CAD build for the part. Positions are in the model's coordinates, mm. Face numbers are marked on the shaded views. A direction names the side the tool comes from. Give positions to 0.01 mm unless a question says otherwise; leave off trailing zeros. Order: outer loops, then holes, each group sorted by start corner. A loop starts at its lowest first (then second) coordinate and runs counter-clockwise, first axis right, second up. Notation, with made-up numbers: (44.5, 52) -> (62.5, 52) arc R33 ccw to (62.5, 84) -> close; hole circle Ø4 at (29.25, 2). An arc over 180 degrees is marked (long way). Use one line per item in the form item = value. Start each with the question number.
1) Drop flat-ended pins along their axis: P1, Ø12, axis at y = -218.5, z = -138.5, coming from the -X side; P2, Ø8, axis at y = -97.5, z = -104.5, coming from the +X side. Give the stop position or say it passes through.
2) Tool access for the marked faces 4, 5, 6, 7 and 8: list every direction of +Z, -Z, +X, -X, +Y, -Y with a clear straight run to the whole face (end or side of a thin tool).
3) Mould opens along Z. For the marked faces 1, 2 and 3 say: pulls with the +Z half, pulls with the -Z half, needs draft (parallel to the pull), parting line crosses it, or undercut.
4) Cut at C-C, the plane x = -40.5. Give the cut face in (y, z), and give its area (3 significant figures).
5) Probe line 1 (Y direction, x = 0, z = -21); line 2 (X direction, y = -225, z = -160.5); line 3 (Z direction, x = -13, y = -263.5). List the from-to ranges inside material, lowest first.
6) Cut at B-B, the plane y = 0. Give the cut face in (x, z), and give its area (3 significant figures).
7) Cut at A-A, the plane z = -18.5. Give the cut face in (x, y), and give its area (3 significant figures).
8) Cut at D-D, the plane z = -114.3. Give the cut face in (x, y).
Autodesk Inventor part; units mm, degrees
ref_plane "YZ Plane" through (0, 0, 0) normal (1, 0, 0) x (0, 1, 0)
ref_plane "XZ Plane" through (0, 0, 0) normal (0, 1, 0) x (-1, 0, 0)
ref_plane "XY Plane" through (0, 0, 0) normal (0, 0, 1) x (1, 0, 0)
sketch "Sketch1" plane through (0, 0, 0) normal (0, 0, 1) x (1, 0, 0)
  circle A0 centre (0, 0) radius 34.29
  line L0 (-120.65, -78.74) -> (120.65, -78.74)
  line L1 (120.65, -78.74) -> (120.65, 48.26)
  line L2 (90.17, 78.74) -> (-90.17, 78.74)
  line L3 (-120.65, 48.26) -> (-120.65, -78.74)
  arc A1 (-90.17, 78.74) -> (-120.65, 48.26) centre (-90.17, 48.26) ccw
  arc A2 (120.65, 48.26) -> (90.17, 78.74) centre (90.17, 48.26) ccw
  point P0 (120.65, 78.74)
  point P1 (-120.65, 78.74)
  dimension "d0" = 68.58
  dimension "d1" = 157.48
  dimension "d2" = 241.3
  dimension "d3" = 78.74
  dimension "d4" = 120.65
  dimension "d5" = 30.48
extrude "Extrusion1" add sketch "Sketch1" against normal blind 187.96
sketch "Sketch2" plane through (0, 0, -187.96) normal (0, 0, -1) x (-1, 0, 0)
  circle A0 centre (0, 0) radius 34.29
  circle A1 centre (0, 0) radius 52.0012
extrude "Extrusion2" add sketch "Sketch2" against normal blind 101.6 contours A0 | A1
sketch "Sketch3" plane through (-120.65, -78.74, 0) normal (-1, 0, 0) x (0, 0, 1)
  line L0 (-187.96, 0) -> (-187.96, 127)
  line L1 (-187.96, 127) -> (-58.42, 127)
  line L2 (-58.42, -30.48) -> (-58.42, -215.9)
  line L3 (-58.42, -215.9) -> (-187.96, -215.9)
  line L4 (-187.96, -215.9) -> (-187.96, 127)
  line L5 (0, 0) -> (-187.96, 0)
  line L6 (-27.94, 0) -> (0, 0)
  line L7 (-187.96, -215.9) -> (-58.42, -215.9)
  line L8 (-58.42, -215.9) -> (-58.42, -30.48)
  line L9 (-58.42, 0) -> (-187.96, 0)
  line L10 (-187.96, 0) -> (-187.96, -215.9)
  arc A0 (-27.94, 0) -> (-58.42, -30.48) centre (-27.94, -30.48) ccw
  line L11 (0, 0) -> (-187.96, 0)
  line L12 (-187.96, -215.9) -> (-58.42, -215.9)
  arc A1 (-27.94, 0) -> (-58.42, -30.48) centre (-27.94, -30.48) ccw
  line L13 (-58.42, -30.48) -> (-58.42, -215.9)
  line L14 (-187.96, -215.9) -> (-187.96, 0)
  line L15 (-187.96, 0) -> (-27.94, 0)
  arc A2 (-27.94, 0) -> (-58.42, -30.48) centre (-27.94, -30.48) ccw
  point P0 (0, 78.74)
  dimension "d10" = 129.54
  dimension "d11" = 342.9
  dimension "d12" = 30.48
extrude "Extrusion3" add sketch "Sketch3" against normal blind 114.3
fillet "Fillet1" radius 30.48 1 edges at (-6.35, -78.74, -107.95)
sketch "Sketch4" plane through (-120.65, -78.74, 0) normal (-1, 0, 0) x (0, 0, 1)
  line L0 (0, 127) -> (-187.96, 127)
  line L1 (-187.96, 127) -> (-187.96, 69.85)
  line L2 (-187.96, 127) -> (-187.96, 0)
  line L3 (-144.78, 78.74) -> (-114.3, 78.74)
  circle A0 centre (-114.3, 78.74) radius 30.48
  line L4 (0, 127) -> (0, 0)
  point P0 (0, 78.74)
  dimension "d18" = 60.96
  dimension "d17" = 57.15
  dimension "d21" = 114.3
  dimension "d25" = 0
extrude "Extrusion4" add sketch "Sketch4" along normal blind 63.5
sketch "Sketch5" plane through (120.65, -78.74, 0) normal (1, 0, 0) x (0, 0, -1)
  line L0 (-23.8125, -17.4625) -> (228.6, -17.4625)
  line L1 (228.6, -17.4625) -> (228.6, 187.325)
  line L2 (228.6, 187.325) -> (-23.8125, 187.325)
  line L3 (-23.8125, 187.325) -> (-23.8125, -17.4625)
  point P0 (0, 78.74)
extrude "Extrusion5" cut sketch "Sketch5" against normal blind 63.5
fillet "Fillet2" radius 30.48 1 edges at (57.15, 78.74, -93.98)
equation "\"d3\" = 0.5 * d1"
properties part number "Shoulder1 Link-lrg"
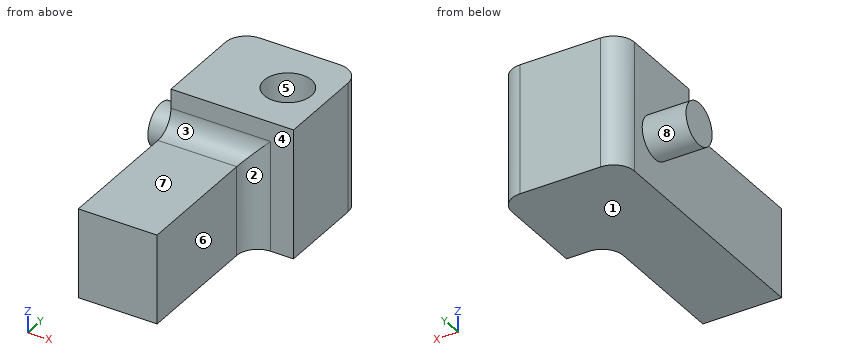
Result:
q1.P1 = -120.65
q1.P2 = -1.98
q2.face_4 = +Z, +X, -Y
q2.face_5 = +Z
q2.face_6 = +Z, -Z, +X, -Y
q2.face_7 = +Z, +X, -X, -Y
q2.face_8 = -X
q3.face_1 = pulls with the -Z half
q3.face_2 = needs draft
q3.face_3 = pulls with the +Z half
q4.outline = (-294.64, -187.96) -> (78.74, -187.96) -> (78.74, 0) -> (-78.74, 0) -> (-78.74, -27.94) arc R30.48 cw to (-109.22, -58.42) -> (-294.64, -58.42) -> close
q4.area = 57,800 mm²
q5.line_1 = -78.74 to -34.29, 34.29 to 78.74
q5.line_2 = -120.65 to -6.35
q5.line_3 = -187.96 to -58.42
q6.outline = (-184.15, -144.78) -> (-120.65, -144.78) -> (-120.65, -187.96) -> (57.15, -187.96) -> (57.15, 0) -> (34.29, 0) -> (34.29, -86.36) -> (-34.29, -86.36) -> (-34.29, 0) -> (-120.65, 0) -> (-120.65, -83.82) -> (-184.15, -83.82) -> close
q6.area = 31,400 mm²
q7.outline = (-120.65, -78.74) -> (57.15, -78.74) -> (57.15, 48.26) arc R30.48 ccw to (26.67, 78.74) -> (-90.17, 78.74) arc R30.48 ccw to (-120.65, 48.26) -> close; hole circle Ø68.58 at (0, 0)
q7.area = 23,900 mm²
q8.outline = (-184.15, -30.48) -> (-120.65, -30.48) -> (-120.65, -294.64) -> (-6.35, -294.64) -> (-6.35, -109.22) arc R30.48 cw to (24.13, -78.74) -> (57.15, -78.74) -> (57.15, 48.26) arc R30.48 ccw to (26.67, 78.74) -> (-90.17, 78.74) arc R30.48 ccw to (-120.65, 48.26) -> (-120.65, 30.48) -> (-184.15, 30.48) -> close
